```python
from build123d import *

# Parameters (mm, degrees)
SKETCH1_R           = 2.75
SKETCH1_W           = 65
SKETCH1_H           = 151
BOSS_EXTRUDE1_DEPTH = 20
SKETCH3_W           = 65
SKETCH3_H           = 151
BOSS_EXTRUDE2_DEPTH = 3.5
SKETCH4_W           = 27.94
SKETCH4_H           = 2.2
CUT_EXTRUDE1_DEPTH  = 117.966875653
FILLET1_R           = 2.5


with BuildPart() as part:
    # Sketch1 → Boss-Extrude1 (new body)
    with BuildSketch(Plane(origin=(0, 0, 0), x_dir=(1, 0, 0), z_dir=(0, 1, 0))):
        with BuildLine():
            Line((-37.5, 75.5), (-37.5, -75.5))
            Line((-37.5, -75.5), (-37.5, -83))
            ThreePointArc((-37.5, -83), (-33, -87.5), (-28.5, -83))
            Line((-28.5, -83), (-28.5, -80.5))
            Line((-28.5, -80.5), (28.5, -80.5))
            Line((28.5, -80.5), (28.5, -83))
            ThreePointArc((28.5, -83), (33, -87.5), (37.5, -83))
            Line((37.5, -83), (37.5, -75.5))
            Line((37.5, -75.5), (37.5, 75.5))
            Line((37.5, 75.5), (37.5, 83))
            ThreePointArc((37.5, 83), (33, 87.5), (28.5, 83))
            Line((28.5, 83), (28.5, 80.5))
            Line((28.5, 80.5), (-28.5, 80.5))
            Line((-28.5, 80.5), (-28.5, 83))
            ThreePointArc((-28.5, 83), (-33, 87.5), (-37.5, 83))
            Line((-37.5, 83), (-37.5, 75.5))
        make_face()
        with Locations(Location((-33, -83, 0), (0, 0, 270))):
            Circle(SKETCH1_R, mode=Mode.SUBTRACT)
        with Locations(Location((33, -83, 0), (0, 0, 90))):
            Circle(SKETCH1_R, mode=Mode.SUBTRACT)
        with Locations(Location((33, 83, 0), (0, 0, 270))):
            Circle(SKETCH1_R, mode=Mode.SUBTRACT)
        with Locations(Location((-33, 83, 0), (0, 0, 90))):
            Circle(SKETCH1_R, mode=Mode.SUBTRACT)
        Rectangle(SKETCH1_W, SKETCH1_H, mode=Mode.SUBTRACT)
    extrude(amount=BOSS_EXTRUDE1_DEPTH)

    # Sketch3 → Boss-Extrude2 (add)
    with BuildSketch(Plane.XZ):
        Rectangle(SKETCH3_W, SKETCH3_H)
    extrude(amount=-BOSS_EXTRUDE2_DEPTH)

    # Sketch4 → Cut-Extrude1 (cut, through all)
    with BuildSketch(Plane.ZY.offset(37.5)):
        with Locations((0, 1.1)):
            Rectangle(SKETCH4_W, SKETCH4_H)
    extrude(amount=-CUT_EXTRUDE1_DEPTH, mode=Mode.SUBTRACT)

    # Fillet1
    fillet1_edges = [part.edges().sort_by_distance(p)[0] for p in [
        (28.5, 10, 80.5),
        (-28.5, 10, 80.5),
        (28.5, 10, -80.5),
        (-28.5, 10, -80.5),
    ]]
    fillet(fillet1_edges, radius=FILLET1_R - 0.0001)  # a hair under: the kernel refuses the full size


solid = part.part
```
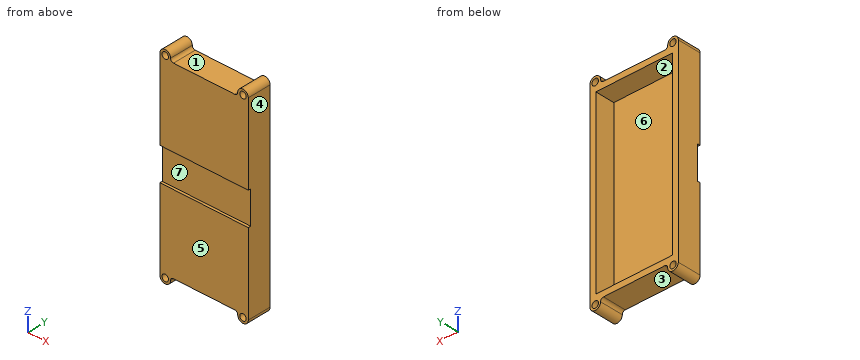
Part model, mm, in its own coordinate system. Face numbers are marked on the shaded views. A direction names the side the tool comes from. Round coordinates to 2 decimals unless told otherwise and drop trailing zeros. Loops run counter-clockwise (first coordinate to the right, second up) from the corner with the lowest first, then second, coordinate; pieces in that order, holes last. Notation, with made-up numbers: (69, 28) -> (118, 28) arc R27 ccw to (118, 57) -> close; hole circle Ø6 at (56.25, 45.5). An arc over 180 degrees is marked (long way). Use one line per item in the form item = value. Start each with the question number.
Item 1: Band-saw the part on A-A (y = 15). Give the number of separate pieces and of enclosed holes in the cut face, plus the area to 3 significant figures.
Item 2: Drop flat-ended pins along their axis: pin 1 Ø1 at (x, y) = (26, 6.5) entering from -Z; pin 2 Ø5 at (x, y) = (3, 11) entering from -Z; pin 3 Ø5 at (x, z) = (-33, 83) entering from +Y; pin 4 Ø1.1 at (x, y) = (0.5, 1) entering from +Z. Give the stop position or say it passes through.
Item 3: Tool access for the marked faces 5, 6 and 7: list every direction of +Z, -Z, +X, -X, +Y, -Y with a clear straight run to the whole face (end or side of a thin tool).
Item 4: Band-saw the part on C-C (z = -67). List the corners of the cut face in (x, y), plus the area to 4 significant figures.
Item 5: Band-saw the part on B-B (x = -8). List the corners of the cut face in (y, z).
Item 6: Drill centre lines: line 1 along X through (y, z) = (10.5, 83); line 2 along X through (y, z) = (8, 58.5); line 3 along Z through (x, y) = (22, 13.5). Where is each one in solid material? Low to high.
Item 7: Two-plate mould, pull along Z, no slides. Class the marked faces 1, 2, 3 and 4: released by +Z, released by -Z, zero draft, split by the parting line, or undercut.
Data:
q1.separate_pieces = 1
q1.enclosed_holes = 5
q1.area = 2,390 mm^2
q2.pin_1 = -80.55
q2.pin_2 = -80.5
q2.pin_3 = through
q2.pin_4 = 80.5
q3.face_5 = +Z, -Z, +X, -X, -Y
q3.face_6 = +Y
q3.face_7 = +X, -X, -Y
q4.outline = (-37.5, 0) -> (37.5, 0) -> (37.5, 20) -> (32.5, 20) -> (32.5, 3.5) -> (-32.5, 3.5) -> (-32.5, 20) -> (-37.5, 20) -> close
q4.area = 427.5 mm^2
q5.outline = (0, -80.5) -> (20, -80.5) -> (20, -75.5) -> (3.5, -75.5) -> (3.5, 75.5) -> (20, 75.5) -> (20, 80.5) -> (0, 80.5) -> (0, 13.97) -> (2.2, 13.97) -> (2.2, -13.97) -> (0, -13.97) -> close
q6.line_1 = -37.5 to -35.75, -30.25 to -28.5, 28.5 to 30.25, 35.75 to 37.5
q6.line_2 = -37.5 to -32.5, 32.5 to 37.5
q6.line_3 = -80.5 to -75.5, 75.5 to 80.5
q7.face_1 = released by +Z
q7.face_2 = undercut
q7.face_3 = released by -Z
q7.face_4 = zero draft
